Verification items for this drawing (mm, ordinates from the low corner). Round coordinates to 2 decimals unless told otherwise and drop trailing zeros. Write each loop counter-clockwise with the first axis right and the second up, starting at its lowest first coordinate (ties: lowest second). Pieces come first, ordered by that corner, then holes. Notation, with made-up numbers: (18.5, -32) -> (56.5, -32) arc R25 ccw to (56.5, -13) -> close; hole circle Ø2 at (10, 41). An arc over 180 degrees is marked (long way). One line per item, written item: value.
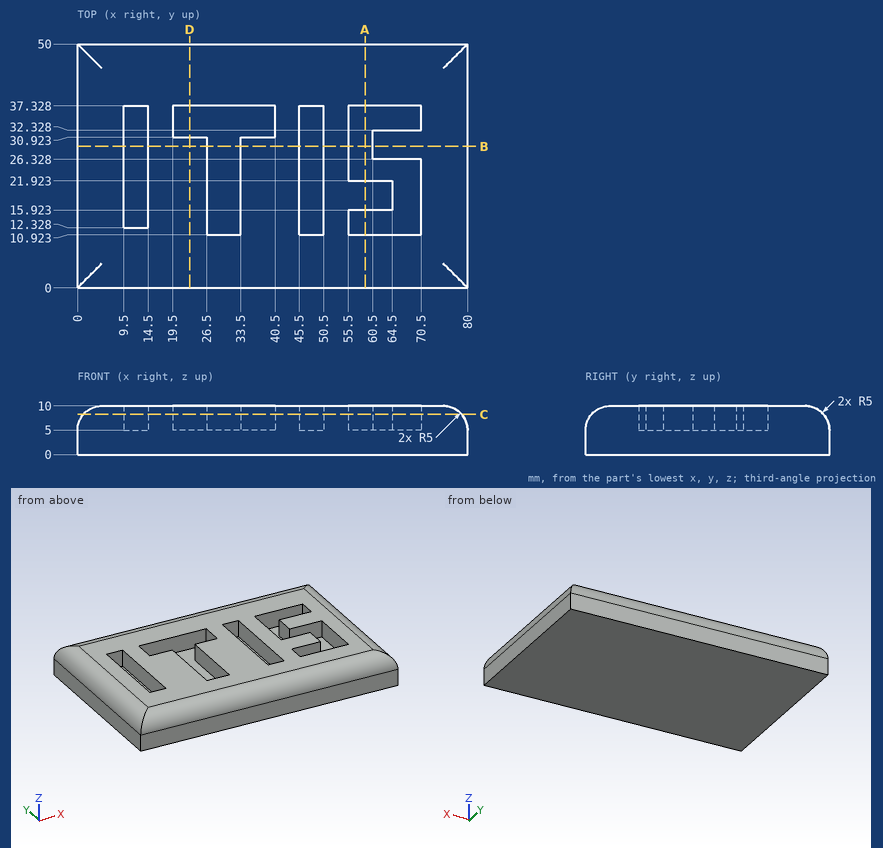
Item 1: Sectioned sample at A-A (x = 59). Enter the section's corners in (y, z).
Result set:
outline: (0, 0) -> (50, 0) -> (50, 5) arc R5 ccw to (45, 10) -> (37.33, 10) -> (37.33, 5) -> (21.92, 5) -> (21.92, 10) -> (15.92, 10) -> (15.92, 5) -> (10.92, 5) -> (10.92, 10) -> (5, 10) arc R5 ccw to (0, 5) -> close
Item 2: Sectioned sample at C-C (z = 8.25). State how many separate pieces and enclosed holes the cut face has, then the cut area to 3 significant figures.
Result set:
separate pieces: 1
enclosed holes: 4
area: 2,880 mm^2
Item 3: Material ranges on line 1 along Z through (x, y) = (57, 30); line 2 along X through (y, z) = (30, 6); line 3 along Y through (x, z) = (10.5, 5.5) (1 decimal), recorded low to high.
Result set:
line 1: 0 to 5
line 2: 0.1 to 9.5, 14.5 to 26.5, 33.5 to 45.5, 50.5 to 55.5, 60.5 to 79.9
line 3: 0 to 12.3, 37.3 to 50
Item 4: Sectioned sample at B-B (y = 29). Enter the section's corners in (x, z).
Result set:
outline: (0, 0) -> (80, 0) -> (80, 5) arc R5 ccw to (75, 10) -> (60.5, 10) -> (60.5, 5) -> (55.5, 5) -> (55.5, 10) -> (50.5, 10) -> (50.5, 5) -> (45.5, 5) -> (45.5, 10) -> (33.5, 10) -> (33.5, 5) -> (26.5, 5) -> (26.5, 10) -> (14.5, 10) -> (14.5, 5) -> (9.5, 5) -> (9.5, 10) -> (5, 10) arc R5 ccw to (0, 5) -> close
Item 5: Depth check by flat-ended pin: pin 1 (5.5 mm diameter, centred on x = 23, z = 8, fed in from +Y); pin 2 (4 mm diameter, centred on y = 30.5, z = 8, fed in from -X); pin 3 (4 mm diameter, centred on x = 62.5, z = 8.5, fed in from +Y). Enter the tip coordinate at first touch or a pass-through.
Result set:
pin 1: y = 49.99
pin 2: x = 0.1
pin 3: y = 49.77
Item 6: Sectioned sample at D-D (x = 23). Enter the section's corners in (y, z), then the cut area to 3 significant figures.
Result set:
outline: (0, 0) -> (50, 0) -> (50, 5) arc R5 ccw to (45, 10) -> (37.33, 10) -> (37.33, 5) -> (30.92, 5) -> (30.92, 10) -> (5, 10) arc R5 ccw to (0, 5) -> close
area: 457 mm^2
